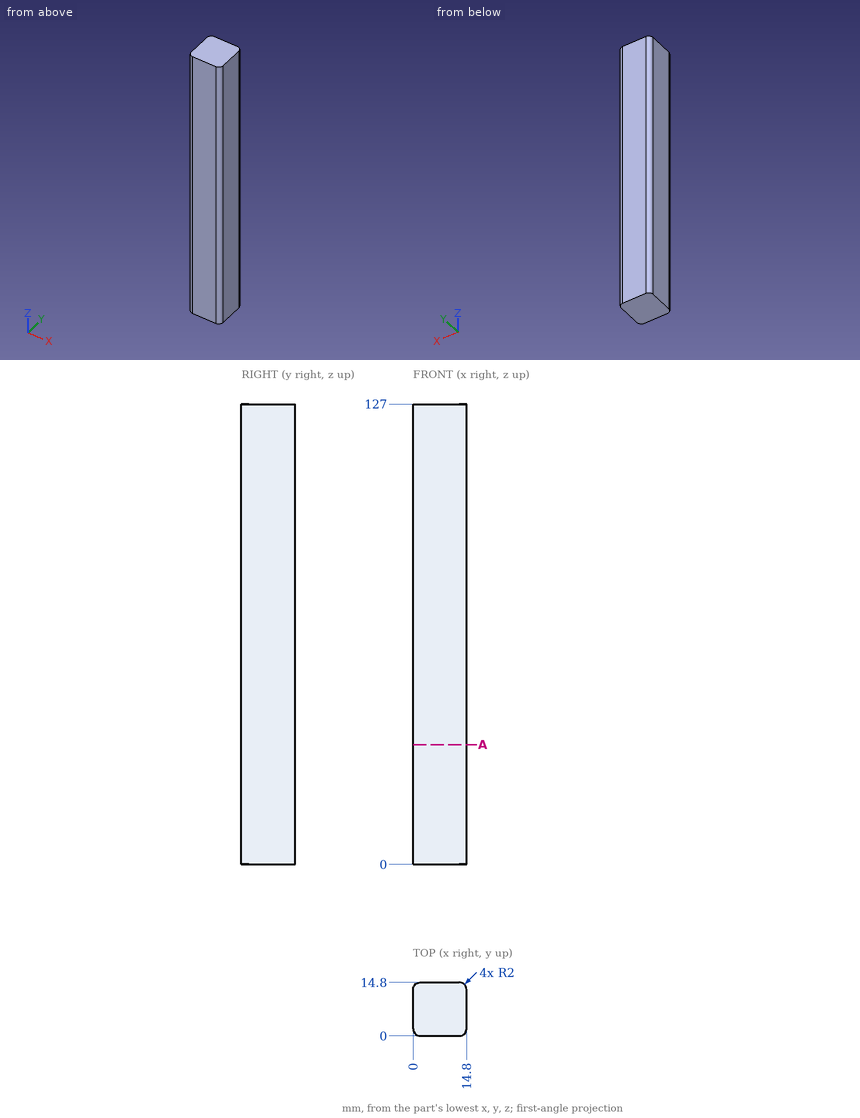
Check sheet for the drawn part. Datum: minimum x, y, z corner. Units: mm. Coordinates: 2 decimals unless noted, no trailing zeros. Loops run counter-clockwise (first coordinate to the right, second up) from the corner with the lowest first, then second, coordinate; pieces in that order, holes last. Notation, with made-up numbers: (35, 8) -> (59, 8) arc R6 cw to (59, 19) -> close; hole circle Ø10 at (6.5, 13). An arc over 180 degrees is marked (long way). Answer as a JSON object with one key per item and string values. Group by question number.
Item 1: Sectioned sample at A-A on z = 33. Record the boundary of the cut face in (x, y).
Item 2: Depth check by flat-ended pin: pin 1 (1.5 mm diameter, centred on x = 5, z = 114, fed in from -Y). Enter the tip coordinate at first touch or a pass-through.
Item 3: Scan lines: probe 1 along X at (y, z) = (13, 40); probe 2 along Y at (x, z) = (1, 64); probe 3 along X at (y, z) = (13.25, 77.5). Record each from-to range of solid material in increasing order.
Evaluation:
{
 "1": {"outline": "(0, 2) arc R2 ccw to (2, 0) -> (12.8, 0) arc R2 ccw to (14.8, 2) -> (14.8, 12.8) arc R2 ccw to (12.8, 14.8) -> (2, 14.8) arc R2 ccw to (0, 12.8) -> close"},
 "2": {"pin 1": "stops at y = 0"},
 "3": {"probe 1": "x = 0.01 to 14.79", "probe 2": "y = 0.27 to 14.53", "probe 3": "x = 0.05 to 14.75"}
}
